CAD build for the part. Positions are in the model's coordinates, mm. A direction names the side the tool comes from. Coordinates: 2 decimals unless noted, no trailing zeros. Order: outer loops, then holes, each group sorted by start corner. A loop starts at its lowest first (then second) coordinate and runs counter-clockwise, first axis right, second up.
Autodesk Inventor part; units mm, degrees
ref_plane "YZ Plane" through (0, 0, 0) normal (1, 0, 0) x (0, 1, 0)
ref_plane "XZ Plane" through (0, 0, 0) normal (0, 1, 0) x (-1, 0, 0)
ref_plane "XY Plane" through (0, 0, 0) normal (0, 0, 1) x (1, 0, 0)
sketch "Sketch1" plane through (0, 0, 0) normal (0, 1, 0) x (-1, 0, 0)
  circle A0 centre (0, 0) radius 27.94
  dimension "d0" = 55.88
extrude "Extrusion1" add sketch "Sketch1" along normal blind 5.08
sketch "Sketch6" plane through (0, 5.08, 0) normal (0, 1, 0) x (1, 0, 0)
  circle A0 centre (0, 23.8125) radius 1.9939
  circle A1 centre (20.6222, 11.9063) radius 1.9939
  circle A2 centre (20.6222, -11.9063) radius 1.9939
  circle A3 centre (0, -23.8125) radius 1.9939
  circle A4 centre (-20.6222, -11.9063) radius 1.9939
  circle A5 centre (-20.6222, 11.9063) radius 1.9939
  point P0 (0, 0)
  point P1 (0, 0)
extrude "Extrusion5" cut sketch "Sketch6" against normal blind 25.4
sketch "Sketch12" plane through (0, 5.08, 0) normal (0, 1, 0) x (1, 0, 0)
  circle A0 centre (0, 0) radius 27.94
  line L0 (2.9329, 0) -> (1.4665, -2.54)
  line L1 (1.4665, -2.54) -> (-1.4665, -2.54)
  line L2 (-1.4665, -2.54) -> (-2.9329, 0)
  line L3 (-2.9329, 0) -> (-1.4665, 2.54)
  line L4 (-1.4665, 2.54) -> (1.4665, 2.54)
  line L5 (1.4665, 2.54) -> (2.9329, 0)
  circle A1 centre (-8, 0) radius 1.245
  circle A2 centre (8, 0) radius 1.245
  circle A3 centre (0, 8) radius 1.5
  circle A4 centre (0, -8) radius 1.5
  point P0 (0, 0)
  dimension "d33" = 5.08
extrude "Extrusion9" cut sketch "Sketch12" against normal blind 25.4 contours L0 L1 L2 L3 L4 L5 | A1 | A2 | A3 | A4
properties part number "WheelMount_v2_vCAD"
1) Slice it at A-A (z = 8). List the corners of the cut face in (x, y), plus the area to 3 significant figures.
2) Slice it at B-B (y = 2.25). Give the number of separate pieces and of enclosed holes in the cut face, plus the area to 3 significant figures.
3) Pin check, flat tips, straight feed: P1, Ø2.5, axis at x = -0.5, y = 2, coming from the -Z side; P2, Ø1.5, axis at x = 0, y = 3, coming from the +Z side; P3, Ø1.5, axis at x = -18, y = 1, coming from the +Z side. Stop position of each tip, or through.
4) Which spindle directions (+Z, -Z, +X, -X, +Y, -Y) get a long thin tool onto all of the face, cutting with end or side? Do faces 4 (the flat face through (-6, 0, 0)), 5 (the flat face through (0, 3, 2.54)). Say none if no direction does.
5) Two-plate mould, pull along Z, no slides. Class faces 1 (the flat face through (-6, 5.08, 0)), 2 (the cylindrical face through (3.64, 2.5, -27.7)), 3 (the cylindrical face through (-6.81, 2.58, -0.37)): released by +Z, released by -Z, zero draft, split by the parting line, or undercut.
6) Slice it at C-C (x = 8). List the corners of the cut face in (y, z) (3 decimals), plus the area to 3 significant figures.
7) Drill centre lines: probe 1 along Z at (x, y) = (0, 3.1); probe 2 along X at (y, z) = (4.25, 11.5); probe 3 along X at (y, z) = (2.1, 13.5). Where is each one in solid material? Low to high.
8) Slice it at D-D (x = -23.5). List the corners of the cut face in (y, z), plus the area to 3 significant figures.
Worked out:
1. outline: (-26.77, 0) - (-1.5, 0) - (-1.5, 5.08) - (-26.77, 5.08) - close; (1.5, 0) - (26.77, 0) - (26.77, 5.08) - (1.5, 5.08) - close
1. area: 257 mm2
2. separate pieces: 1
2. enclosed holes: 11
2. area: 2,330 mm2
3. P1: stops at z = -27.94
3. P2: stops at z = 27.94
3. P3: stops at z = 21.98
4. face 4: +Z, -Z, +X, -X, -Y
4. face 5: +Y, -Y
5. face 1: zero draft
5. face 2: split by the parting line
5. face 3: undercut
6. outline: (0, -26.77) - (5.08, -26.77) - (5.08, -1.245) - (0, -1.245) - close; (0, 1.245) - (5.08, 1.245) - (5.08, 26.77) - (0, 26.77) - close
6. area: 259 mm2
7. probe 1: z = -27.94 to -25.81, -21.82 to -9.5, -6.5 to -2.54, 2.54 to 6.5, 9.5 to 21.82, 25.81 to 27.94
7. probe 2: x = -25.46 to -22.57, -18.67 to 18.67, 22.57 to 25.46
7. probe 3: x = -24.46 to -21.82, -19.42 to 19.42, 21.82 to 24.46
8. outline: (0, -15.11) - (5.08, -15.11) - (5.08, 15.11) - (0, 15.11) - close
8. area: 154 mm2
